Study the drawing (mm; zero at the part's minimum x, y, z) and answer. A direction names the side the tool comes from. Round coordinates to 2 decimals unless told otherwise and drop trailing zeros. Loops run counter-clockwise (first coordinate to the right, second up) from the corner with the lowest first, then second, coordinate; pieces in that order, holes last. Notation, with made-up numbers: (-2.5, -34.75) -> (40.5, -34.75) arc R28 cw to (40.5, -15.75) -> close; hole circle Ø8 at (79, 49). An arc over 180 degrees is marked (long way). Write each question's results on one line, items separated by ' | '. Start each with the question number.
(1) For the marked faces 4 and 5, determine the directions among +Z, -Z, +X, -X, +Y, -Y from which every point of the face is accessible in a straight line to the end or side of a thin tool.
(2) The part is cut by section A-A (x = 26). Determine the outline of the cut face in (y, z), plus the area to 3 significant figures.
(3) The part is cut by section D-D (y = 27). Determine the outline of the cut face in (x, z), plus the area to 3 significant figures.
(4) Straight lines are drawn through the part: probe 1 along X at (y, z) = (19.5, 22.5); probe 2 along Z at (x, y) = (38, 5); probe 3 along X at (y, z) = (25.5, 18.5). For each, find the intervals that lie inside material, in ascending order.
(5) Flat-ended cylindrical pins translate along their axes: pin 1 (12 mm diameter, centred on y = 25, z = 38.5, fed in from +X); pin 2 (1 mm diameter, centred on y = 28, z = 26.5, fed in from +X); pin 3 (5 mm diameter, centred on y = 5, z = 7, fed in from -X); pin 4 (10 mm diameter, centred on x = 26, y = 9.5, fed in from -Z). Find the tip coordinate at first contact, or state that the pin passes through.
(6) Determine the mould class of the marked faces 1, 2 and 3 for opening direction Z: released by +Z, released by -Z, zero draft, split by the parting line, or undercut.
(7) The part is cut by section C-C (y = 8). Determine the outline of the cut face in (x, z).
(8) The part is cut by section B-B (z = 26). Determine the outline of the cut face in (x, y).
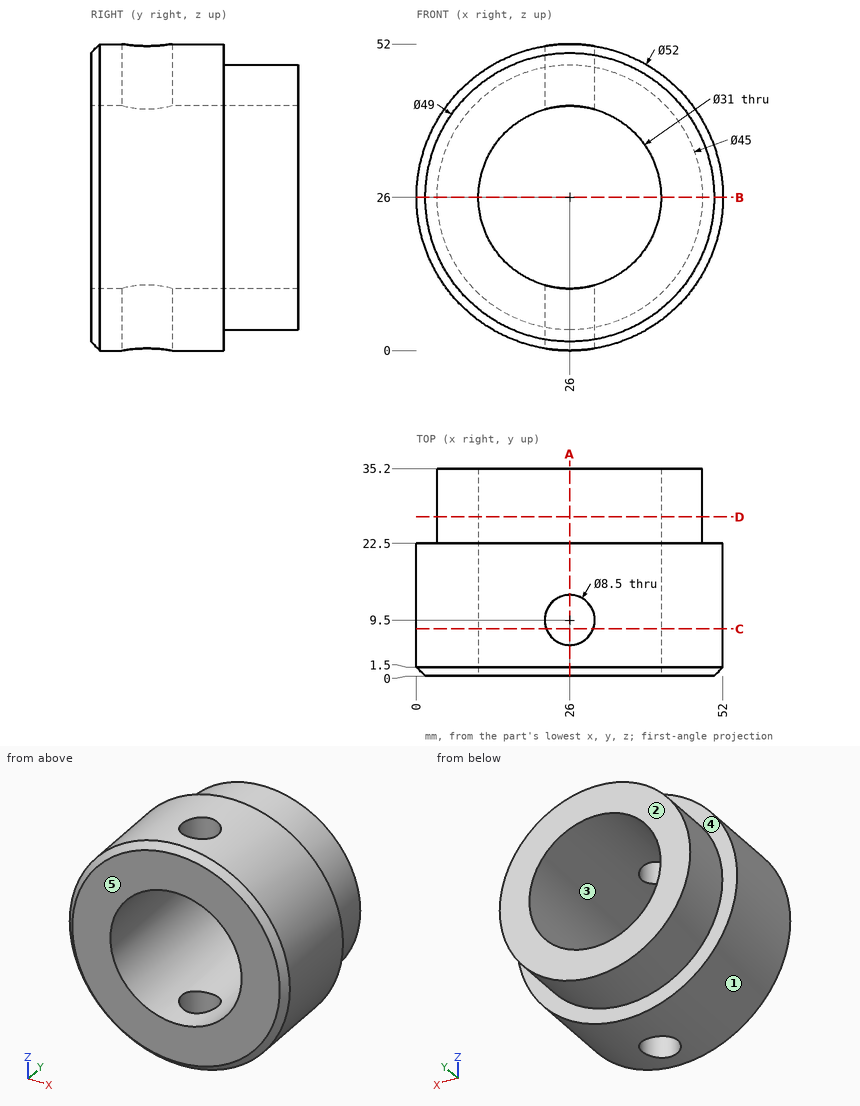
Checked values:
1) face 4: +Y | face 5: +Z, -Z, +X, -X, -Y
2) outline: (0, 1.5) -> (1.5, 0) -> (5.25, 0) -> (5.25, 10.5) -> (0, 10.5) -> close; (0, 41.5) -> (5.25, 41.5) -> (5.25, 52) -> (1.5, 52) -> (0, 50.5) -> close; (13.75, 0) -> (22.5, 0) -> (22.5, 3.5) -> (35.2, 3.5) -> (35.2, 10.5) -> (13.75, 10.5) -> close; (13.75, 41.5) -> (35.2, 41.5) -> (35.2, 48.5) -> (22.5, 48.5) -> (22.5, 52) -> (13.75, 52) -> close | area: 470 mm2
3) outline: circle Ø45 at (26, 26); hole circle Ø31 at (26, 26) | area: 836 mm2
4) probe 1: x = 0.24 to 10.9, 41.1 to 51.76 | probe 2: z = 2.93 to 16.19, 35.81 to 49.07 | probe 3: x = 4.79 to 12.44, 39.56 to 47.21
5) pin 1: stops at x = 51.03 | pin 2: stops at x = 48.5 | pin 3: stops at x = 5.91 | pin 4: stops at z = 0
6) face 1: split by the parting line | face 2: zero draft | face 3: undercut
7) outline: (22.02, 0.31) -> (22.02, 11.02) arc R15.5 cw to (22.02, 40.98) -> (22.02, 51.69) arc R26 ccw to start; (29.98, 0.31) arc R26 ccw to (29.98, 51.69) -> (29.98, 40.98) arc R15.5 cw to (29.98, 11.02) -> close
8) outline: (0, 1.5) -> (1.5, 0) -> (10.5, 0) -> (10.5, 35.2) -> (3.5, 35.2) -> (3.5, 22.5) -> (0, 22.5) -> close; (41.5, 0) -> (50.5, 0) -> (52, 1.5) -> (52, 22.5) -> (48.5, 22.5) -> (48.5, 35.2) -> (41.5, 35.2) -> close
